Can you work these out from the model? Positions are in its coordinate system, mm. Coordinates: 2 decimals unless noted, no trailing zeros. Loops run counter-clockwise (first coordinate to the right, second up) from the corner with the lowest first, then second, coordinate; pieces in that order, holes last. Notation, with made-up numbers: M -10,-5 L 24,-5 A9 cw 24,11 Z; hole C 72,14 d6. An arc over 180 degrees is marked long. Answer as a JSON object with one key per item and string values. Group by question number.
Item 1: Suppose I cut it at B-B (z = -25.5). Write out the boundary of the cut face in (x, y).
Item 2: Suppose I cut it at D-D (y = -3.25). Write out the boundary of the cut face in (x, z), then the cut area to 3 significant figures.
Item 3: If I drill on line 1 (Z direction, x = 0, y = 1.6); line 2 (Z direction, x = 0, y = -1.6); line 3 (X direction, y = 1.5, z = -15), over which ranges is the centre line in solid material (lowest first)?
Item 4: Suppose I cut it at C-C (z = 16). Write out the boundary of the cut face in (x, y).
Item 5: I'm going to push a flat-ended pin straight in: pin 1 Ø3 at (x, y) = (-17.5, 0.5) entering from +Z. Where does the tip first touch, or does it pass through?
Item 6: Suppose I cut it at A-A (x = 0). Write out the boundary of the cut face in (y, z).
```python
from build123d import *

# Parameters (mm, degrees)
SKETCH1_W                = 88
SKETCH1_H                = 88
BOSS_EXTRUDE1_DEPTH      = 2
FILLET1_R                = 10
SKETCH3_R                = 37
CUT_EXTRUDE2_DEPTH       = 3
SKETCH5_R                = 40.5
SKETCH5_R_2              = 10
BOSS_EXTRUDE2_DEPTH      = 2
CUT_EXTRUDE3_DEPTH       = 3
CIRPATTERN1_COUNT        = 3
SKETCH17_R               = 27.977706125
CUT_EXTRUDE4_DEPTH       = 3
CUT_EXTRUDE5_DEPTH       = 3
FILLET2_R                = 2
SKETCH19_R               = 13.2
SKETCH19_R_2             = 8.2
BOSS_EXTRUDE3_DEPTH      = 5
BOSS_EXTRUDE3_DEPTH_BACK = 2
SKETCH20_R               = 1.6
CUT_EXTRUDE6_DEPTH       = 3
CIRPATTERN2_COUNT        = 3


with BuildPart() as part:
    # Sketch1 → Boss-Extrude1 (new body)
    with BuildSketch(Plane(origin=(0, 0, 0), x_dir=(1, 0, 0), z_dir=(0, 1, 0))):
        Rectangle(SKETCH1_W, SKETCH1_H)
    extrude(amount=BOSS_EXTRUDE1_DEPTH)

    # Fillet1
    fillet1_edges = [part.edges().sort_by_distance(p)[0] for p in [
        (44, 1, 44),
        (-44, 1, 44),
        (-44, 1, -44),
        (44, 1, -44),
    ]]
    fillet(fillet1_edges, radius=FILLET1_R)

    # Sketch3 → Cut-Extrude2 (cut, through all)
    with BuildSketch(Plane(origin=(0, 2, 0), x_dir=(1, 0, 0), z_dir=(0, 1, 0))):
        Circle(SKETCH3_R)
    extrude(amount=-CUT_EXTRUDE2_DEPTH, mode=Mode.SUBTRACT)

    # Sketch5 → Boss-Extrude2 (add)
    with BuildSketch(Plane(origin=(0, 0, 0), x_dir=(1, 0, 0), z_dir=(0, 1, 0))):
        Circle(SKETCH5_R)
        Circle(SKETCH5_R_2, mode=Mode.SUBTRACT)
    extrude(amount=BOSS_EXTRUDE2_DEPTH)

    # Sketch16 → Cut-Extrude3 (cut, through all)
    with BuildSketch(Plane(origin=(0, 2, 0), x_dir=(1, 0, 0), z_dir=(0, 1, 0))):
        with BuildLine():
            ThreePointArc((12.654745303, 34.768626969), (13.077619626, 7.550367211), (36.437886861, -6.424982574))
            ThreePointArc((36.437886861, -6.424982574), (32.04293994, 18.5), (12.654745303, 34.768626969))
        make_face()
    cut_extrude3 = extrude(amount=-CUT_EXTRUDE3_DEPTH, mode=Mode.SUBTRACT)

    # CirPattern1: Cut-Extrude3 ×3 about axis
    cirpattern1_axis = Axis((0, 0, 0), (0, 1, 0))
    for i in range(1, CIRPATTERN1_COUNT):
        add(cut_extrude3.rotate(cirpattern1_axis, i * 360 / CIRPATTERN1_COUNT), mode=Mode.SUBTRACT)

    # Sketch17 → Cut-Extrude4 (cut, through all)
    with BuildSketch(Plane(origin=(0, 2, 0), x_dir=(1, 0, 0), z_dir=(0, 1, 0))):
        with Locations((0, -43.078440548)):
            Circle(SKETCH17_R)
    extrude(amount=-CUT_EXTRUDE4_DEPTH, mode=Mode.SUBTRACT)

    # Sketch18 → Cut-Extrude5 (cut, through all)
    with BuildSketch(Plane(origin=(0, 2, 0), x_dir=(1, 0, 0), z_dir=(0, 1, 0))):
        with BuildLine():
            ThreePointArc((-10, 0), (-12.516559025, -12.564476209), (-19.677986964, -23.190532939))
            ThreePointArc((-19.677986964, -23.190532939), (0, -15.100734422), (19.677986964, -23.190532939))
            ThreePointArc((19.677986964, -23.190532939), (12.516559025, -12.564476209), (10, 0))
            ThreePointArc((10, 0), (0, -10), (-10, 0))
        make_face()
    extrude(amount=-CUT_EXTRUDE5_DEPTH, mode=Mode.SUBTRACT)

    # Fillet2
    fillet2_edges = [part.edges().sort_by_distance(p)[0] for p in [
        (-27.962524354, 1, 44),
        (27.962524354, 1, 44),
    ]]
    fillet(fillet2_edges, radius=FILLET2_R)

    # Sketch19 → Boss-Extrude3 (add, two sides)
    with BuildSketch(Plane.XZ) as boss_extrude3_sk:
        Circle(SKETCH19_R)
        Circle(SKETCH19_R_2, mode=Mode.SUBTRACT)
    extrude(amount=BOSS_EXTRUDE3_DEPTH)
    extrude(boss_extrude3_sk.sketch, amount=-BOSS_EXTRUDE3_DEPTH_BACK)

    # Sketch20 → Cut-Extrude6 (cut, through all)
    with BuildSketch(Plane.XZ):
        with Locations((0, -32)):
            Circle(SKETCH20_R)
    cut_extrude6 = extrude(amount=-CUT_EXTRUDE6_DEPTH, mode=Mode.SUBTRACT)

    # CirPattern2: Cut-Extrude6 ×3 about axis
    cirpattern2_axis = Axis((0, 0, 0), (0, 1, 0))
    for i in range(1, CIRPATTERN2_COUNT):
        add(cut_extrude6.rotate(cirpattern2_axis, i * 360 / CIRPATTERN2_COUNT), mode=Mode.SUBTRACT)


solid = part.part
```
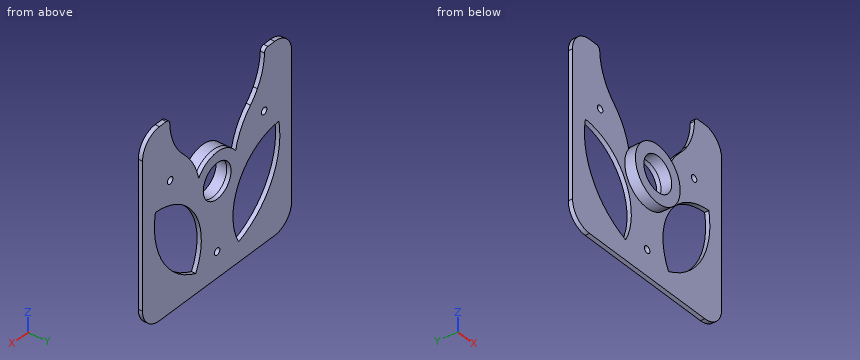
From the geometry:
{
 "1": {"outline": "M -44,0 L -26.81,0 L -26.81,2 L -44,2 Z; M -9.61,0 L 9.61,0 L 9.61,2 L -9.61,2 Z; M 26.81,0 L 44,0 L 44,2 L 26.81,2 Z"},
 "2": {"outline": "C 0,0 d26.4; hole C 0,0 d16.4", "area": "336 mm2"},
 "3": {"line 1": "-44 to -33.6, -30.4 to -8.2, 8.2 to 13.2", "line 2": "-13.2 to -8.2, 8.2 to 13.2", "line 3": "-44 to -33.82, -10.1 to 10.1, 33.82 to 44"},
 "4": {"outline": "M -44,0 L -29.31,0 L -29.31,2 L -44,2 Z; M -26.11,0 L -14.19,0 L -14.19,2 L -26.11,2 Z; M 14.19,0 L 26.11,0 L 26.11,2 L 14.19,2 Z; M 29.31,0 L 44,0 L 44,2 L 29.31,2 Z"},
 "5": {"pin 1": "z = 22.5"},
 "6": {"outline": "M -5,-13.2 L 0,-13.2 L 0,-30.4 L 2,-30.4 L 2,-8.2 L -5,-8.2 Z; M -5,8.2 L 2,8.2 L 2,13.2 L -5,13.2 Z; M 0,-44 L 2,-44 L 2,-33.6 L 0,-33.6 Z"}
}
